Source: CAD feature listing. Evaluate the final solid. Frame: model axes, mm. A direction names the side the tool comes from. Round coordinates to 2 decimals unless told otherwise and drop trailing zeros. Write each loop counter-clockwise with the first axis right and the second up, starting at its lowest first coordinate (ties: lowest second). Pieces come first, ordered by that corner, then holes. Notation, with made-up numbers: M -27.75,5.25 L -11.75,5.25 A20 ccw -11.75,22.25 Z; hole C 62.5,-8 d9. An arc over 180 degrees is marked long. Answer in a Markdown table with one row per item. Add a question column.
Item 1: Contact query for flat-ended pins moving along their axis: pin 1 (8 mm diameter, centred on x = -40, z = -40, fed in from +Y); pin 2 (1.5 mm diameter, centred on x = 12, y = 27, fed in from +Z); pin 3 (22.5 mm diameter, centred on y = 41, z = -3.5, fed in from -X); pin 4 (11.5 mm diameter, centred on x = 40, z = -40, fed in from +Y). Output: stop coordinate, or through.
Item 2: Set-up query: faces 4 (the face through (-24.181, 74.93, 23.902)), 5 (the face through (-10, 35, 34)), 6 (the face through (-23.902, 34.65, -24.181)). Return all of +Z, -Z, +X, -X, +Y, -Y with unobstructed straight access to the full face (end or side cutting, diameter ignored); none if empty.
Item 3: Cut plane A-A on y = 35. Return loops of the section in (x, z).
Item 4: Cut plane B-B on z = 0. Return loops of the section in (x, y), and give its area (3 significant figures).
Item 5: Cut plane C-C on y = 67.5. Return loops of the section in (x, z).
Item 6: Mould query, pull axis Z, two halves, no side actions, for faces 1 (the face through (-23.902, 74.93, -24.181)), 2 (the face through (43, 5, 44)), 3 (the face through (-50, 5, -1)). Classes: released by +Z, released by -Z, zero draft, split by the parting line, or undercut.
Item 7: Cut plane D-D on y = 23.5. Return loops of the section in (x, z), and give its area (3 significant figures).
Item 8: Material intervals for probe 1 along X at (y, z) = (3.75, 40); probe 2 along Y at (x, z) = (-28.5, 39.5); probe 3 along X at (y, z) = (72, 0), sorted ascending.
from build123d import *

# Parameters (mm, degrees)
BOSS_EXTRUDE1_DEPTH = 80
SKETCH2_R           = 25
CUT_EXTRUDE1_DEPTH  = 10
SKETCH3_R           = 15
CUT_EXTRUDE2_DEPTH  = 70
SKETCH4_R           = 5
BOSS_EXTRUDE2_DEPTH = 10
SKETCH5_R           = 5
BOSS_EXTRUDE3_DEPTH = 10
SKETCH6_R           = 15
CUT_EXTRUDE3_DEPTH  = 80
SKETCH7_R           = 9
CUT_EXTRUDE4_DEPTH  = 80


with BuildPart() as part:
    # Sketch1 → Boss-Extrude1 (new body)
    with BuildSketch(Plane(origin=(0, 0, 0), x_dir=(1, 0, 0), z_dir=(0, 1, 0))):
        Polygon((34, 14.083261121), (14.083261121, 34), (-14.083261121, 34), (-34, 14.083261121), (-34, -14.083261121), (-14.083261121, -34), (14.083261121, -34), (34, -14.083261121), align=None)
    extrude(amount=BOSS_EXTRUDE1_DEPTH)

    # Sketch2 → Cut-Extrude1 (cut)
    with BuildSketch(Plane(origin=(0, 80, 0), x_dir=(1, 0, 0), z_dir=(0, 1, 0))):
        with Locations(Location((0, 0, 0), (0, 0, 270))):
            Circle(SKETCH2_R)
    extrude(amount=-CUT_EXTRUDE1_DEPTH, mode=Mode.SUBTRACT)

    # Sketch3 → Cut-Extrude2 (cut)
    with BuildSketch(Plane.XZ):
        with Locations(Location((0, 0, 0), (0, 0, 270))):
            Circle(SKETCH3_R)
    extrude(amount=-CUT_EXTRUDE2_DEPTH, mode=Mode.SUBTRACT)

    # Sketch4 → Boss-Extrude2 (add)
    with BuildSketch(Plane.XZ):
        with BuildLine():
            Line((-40, 50), (40, 50))
            ThreePointArc((40, 50), (47.071067812, 47.071067812), (50, 40))
            Line((50, 40), (50, -40))
            ThreePointArc((50, -40), (47.071067812, -47.071067812), (40, -50))
            Line((40, -50), (-40, -50))
            ThreePointArc((-40, -50), (-47.071067812, -47.071067812), (-50, -40))
            Line((-50, -40), (-50, 40))
            ThreePointArc((-50, 40), (-47.071067812, 47.071067812), (-40, 50))
        make_face()
        with Locations(Location((-40, 40, 0), (0, 0, 270))):
            Circle(SKETCH4_R, mode=Mode.SUBTRACT)
        with Locations(Location((40, 40, 0), (0, 0, 270))):
            Circle(SKETCH4_R, mode=Mode.SUBTRACT)
        with Locations(Location((-40, -40, 0), (0, 0, 270))):
            Circle(SKETCH4_R, mode=Mode.SUBTRACT)
        with Locations(Location((40, -40, 0), (0, 0, 270))):
            Circle(SKETCH4_R, mode=Mode.SUBTRACT)
    extrude(amount=-BOSS_EXTRUDE2_DEPTH)

    # Sketch5 → Boss-Extrude3 (add)
    with BuildSketch(Plane(origin=(0, 60, 0), x_dir=(-1, 0, 0), z_dir=(0, -1, 0))):
        with BuildLine():
            Line((-40, 50), (40, 50))
            ThreePointArc((40, 50), (47.071067812, 47.071067812), (50, 40))
            Line((50, 40), (50, -40))
            ThreePointArc((50, -40), (47.071067812, -47.071067812), (40, -50))
            Line((40, -50), (-40, -50))
            ThreePointArc((-40, -50), (-47.071067812, -47.071067812), (-50, -40))
            Line((-50, -40), (-50, 40))
            ThreePointArc((-50, 40), (-47.071067812, 47.071067812), (-40, 50))
        make_face()
        with Locations(Location((-40, 40, 0), (0, 0, 90))):
            Circle(SKETCH5_R, mode=Mode.SUBTRACT)
        with Locations(Location((40, 40, 0), (0, 0, 90))):
            Circle(SKETCH5_R, mode=Mode.SUBTRACT)
        with Locations(Location((-40, -40, 0), (0, 0, 90))):
            Circle(SKETCH5_R, mode=Mode.SUBTRACT)
        with Locations(Location((40, -40, 0), (0, 0, 90))):
            Circle(SKETCH5_R, mode=Mode.SUBTRACT)
    extrude(amount=-BOSS_EXTRUDE3_DEPTH)

    # Sketch6 → Cut-Extrude3 (cut)
    with BuildSketch(Plane.XZ):
        with Locations(Location((0, 0, 0), (0, 0, 270))):
            Circle(SKETCH6_R)
    extrude(amount=-CUT_EXTRUDE3_DEPTH, mode=Mode.SUBTRACT)

    # Sketch7 → Cut-Extrude4 (cut)
    with BuildSketch(Plane.XY.offset(34)):
        with Locations((0, 35)):
            Circle(SKETCH7_R)
    extrude(amount=-CUT_EXTRUDE4_DEPTH, mode=Mode.SUBTRACT)


solid = part.part
Results below:
| question | item | result |
|---|---|---|
| 1 | pin 1 | through |
| 1 | pin 2 | z = 34 |
| 1 | pin 3 | x = -34 |
| 1 | pin 4 | y = 70 |
| 2 | face 4 | +Z, -X, +Y |
| 2 | face 5 | +Z, +X, -X |
| 2 | face 6 | -Z, -X |
| 3 | outline | M -34,-14.08 L -14.08,-34 L -9,-34 L -9,-12 A15 cw -9,12 L -9,34 L -14.08,34 L -34,14.08 Z; M 9,-34 L 14.08,-34 L 34,-14.08 L 34,14.08 L 14.08,34 L 9,34 L 9,12 A15 cw 9,-12 Z |
| 4 | outline | M -50,0 L -15,0 L -15,70 L -25,70 L -25,80 L -34,80 L -34,70 L -50,70 L -50,60 L -34,60 L -34,10 L -50,10 Z; M 15,0 L 50,0 L 50,10 L 34,10 L 34,60 L 50,60 L 50,70 L 34,70 L 34,80 L 25,80 L 25,70 L 15,70 Z |
| 4 | area | 3,480 mm2 |
| 5 | outline | M -50,-40 A10 ccw -40,-50 L 40,-50 A10 ccw 50,-40 L 50,40 A10 ccw 40,50 L -40,50 A10 ccw -50,40 Z; hole C -40,-40 d10; hole C -40,40 d10; hole C 0,0 d30; hole C 40,-40 d10; hole C 40,40 d10 |
| 6 | face 1 | released by -Z |
| 6 | face 2 | undercut |
| 6 | face 3 | zero draft |
| 7 | outline | M -34,-14.08 L -14.08,-34 L 14.08,-34 L 34,-14.08 L 34,14.08 L 14.08,34 L -14.08,34 L -34,14.08 Z; hole C 0,0 d30 |
| 7 | area | 3,120 mm2 |
| 8 | probe 1 | -50 to -45, -35 to 35, 45 to 50 |
| 8 | probe 2 | 0 to 10, 60 to 70 |
| 8 | probe 3 | -34 to -25, 25 to 34 |
